Input: dimensioned drawing with shaded views. Units: mm. Origin: part minimum x, y, z. A direction names the side the tool comes from. Coordinates: 2 decimals unless noted, no trailing zeros. Order: outer loops, then holes, each group sorted by start corner. A loop starts at its lowest first (then second) coordinate and runs counter-clockwise, first axis right, second up. Notation, with made-up numbers: (9, 34) -> (22, 34) arc R26 cw to (22, 51) -> close; hole circle Ø10 at (68.25, -36). An arc over 180 degrees is marked (long way). Put each result on its own line as item: value.
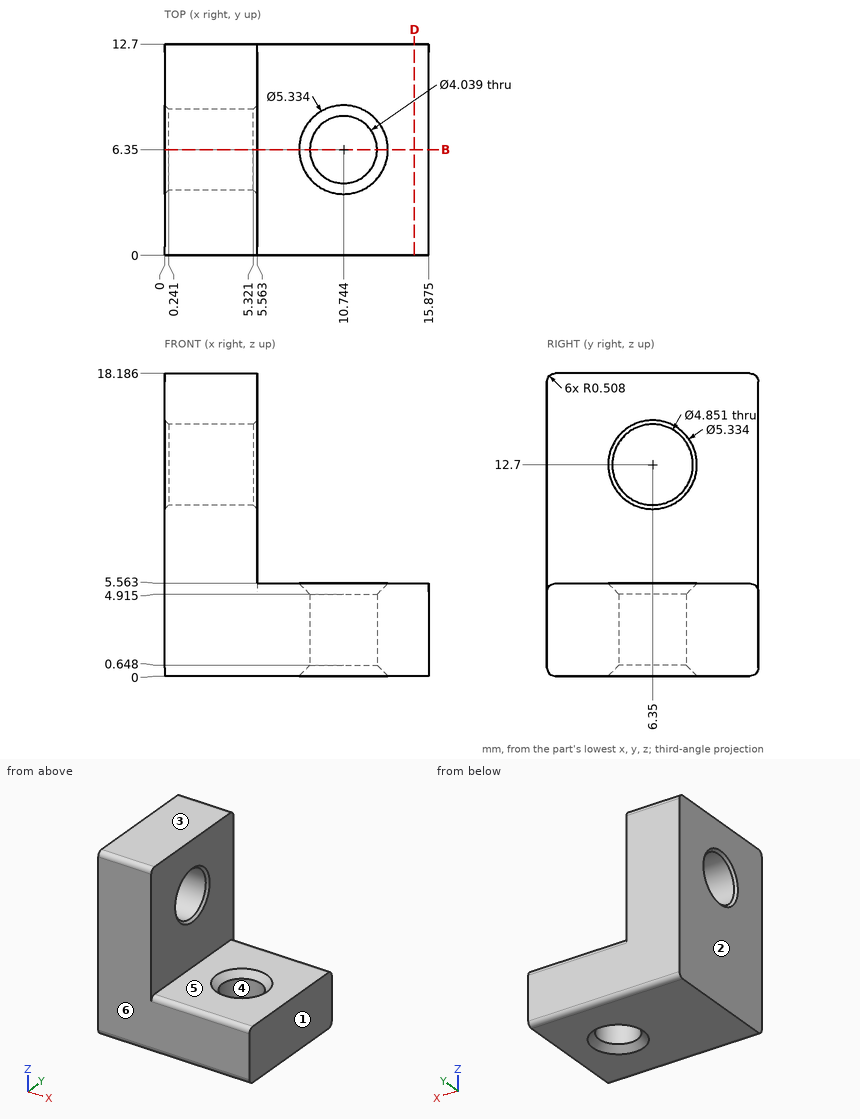
1. Cut plane D-D on x = 15. Output: boundary loops of the cut face in (y, z) (1 decimal).
Numbers:
outline: (0, 0.5) arc R0.5 ccw to (0.5, 0) -> (12.2, 0) arc R0.5 ccw to (12.7, 0.5) -> (12.7, 5.1) arc R0.5 ccw to (12.2, 5.6) -> (0.5, 5.6) arc R0.5 ccw to (0, 5.1) -> close
2. Cut plane B-B on y = 6.35. Count the separate pieces of the cut face and the enclosed holes in it, plus the area to 3 significant figures.
Numbers:
separate pieces: 3
enclosed holes: 0
area: 108 mm2
3. Set-up query: the marked faces 5 and 6. Return all of +Z, -Z, +X, -X, +Y, -Y with unobstructed straight access to the full face (end or side cutting, diameter ignored); none if empty.
Numbers:
face 5: +Z, +X, +Y, -Y
face 6: +Z, -Z, +X, -X, -Y
4. Ray query, line 1 along Z through (x, y) = (1.3, 6.35) (1 decimal); line 2 along X through (y, z) = (6.35, 3.35) (1 decimal); line 3 along Y through (x, z) = (4.2, 12.7) (1 decimal). Return the intervals inside material, ascending.
Numbers:
line 1: z = 0 to 10.3, 15.1 to 18.2
line 2: x = 0 to 8.7, 12.8 to 15.9
line 3: y = 0 to 3.9, 8.8 to 12.7
5. Pull-direction query (X, two-part tool) for the marked faces 1, 2, 3 and 4; classes: pulls with the +X half, pulls with the -X half, needs draft (parallel to the pull), parting line crosses it, or undercut.
Numbers:
face 1: pulls with the +X half
face 2: pulls with the -X half
face 3: needs draft
face 4: undercut
6. First-contact query: pin 1 (3 mm diameter, centred on x = 12, y = 8.5, fed in from +Z); pin 2 (2 mm diameter, centred on x = 10, y = 6, fed in from +Z); pin 3 (1.5 mm diameter, centred on x = 9.5, y = 5.5, fed in from -Z). Flat tips, straight axial feed; report the tip coordinate or a pass-through.
Numbers:
pin 1: stops at z = 5.56
pin 2: passes through
pin 3: stops at z = 0.41
